Build history of the part. All positions in model axes, mm. Face numbers are marked on the shaded views. A direction names the side the tool comes from. Give positions to 0.01 mm unless a question says otherwise; leave off trailing zeros. Write each loop counter-clockwise with the first axis right and the second up, starting at its lowest first coordinate (ties: lowest second). Pieces come first, ordered by that corner, then holes.
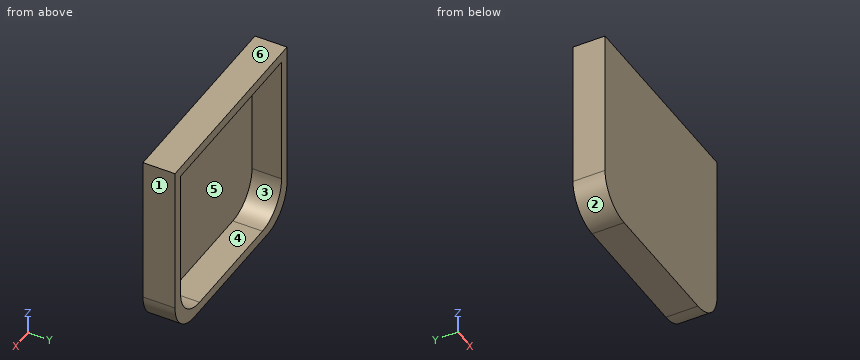
from build123d import *

# Parameters (mm, degrees)
BOSS_EXTRUDE1_DEPTH = 13
CUT_EXTRUDE1_DEPTH  = 12


with BuildPart() as part:
    # Sketch3 → Boss-Extrude1 (new body)
    with BuildSketch(Plane(origin=(0, 0, 0), x_dir=(1, 0, 0), z_dir=(0, 1, 0))):
        with BuildLine():
            Line((-41.015, -37.585), (41.015, -37.585))
            Line((41.015, -37.585), (41.015, 23.585))
            ThreePointArc((41.015, 23.585), (36.914494937, 33.484494937), (27.015, 37.585))
            Line((27.015, 37.585), (-27.015, 37.585))
            ThreePointArc((-27.015, 37.585), (-36.914494937, 33.484494937), (-41.015, 23.585))
            Line((-41.015, 23.585), (-41.015, -37.585))
        make_face()
    extrude(amount=BOSS_EXTRUDE1_DEPTH)

    # Sketch4 → Cut-Extrude1 (cut)
    with BuildSketch(Plane(origin=(0, 13, 0), x_dir=(1, 0, 0), z_dir=(0, 1, 0))):
        with BuildLine():
            Line((-37.015, -33.585), (37.015, -33.585))
            Line((37.015, -33.585), (37.015, 19.585))
            ThreePointArc((37.015, 19.585), (32.914494937, 29.484494937), (23.015, 33.585))
            Line((23.015, 33.585), (-23.015, 33.585))
            ThreePointArc((-23.015, 33.585), (-32.914494937, 29.484494937), (-37.015, 19.585))
            Line((-37.015, 19.585), (-37.015, -33.585))
        make_face()
    extrude(amount=-CUT_EXTRUDE1_DEPTH, mode=Mode.SUBTRACT)


solid = part.part
(1) Saw through at A-A, the plane y = 4.5. List the corners of the cut face in (x, z) (3 decimals), plus the area to 3 significant figures.
(2) Saw through at C-C, the plane z = 2. List the corners of the cut face in (x, y) (3 decimals), plus the area to 3 significant figures.
(3) 3-axis set-ups, long thin cutter, end or side, ignore diameter. For the marked faces 5 and 6: which of +Z, -Z, +X, -X, +Y, -Y reach the whole face in a straight line?
(4) Drop flat-ended pins along their axis: pin 1 (1 mm diameter, centred on x = 15.5, z = -13, fed in from -Y); pin 2 (3 mm diameter, centred on x = 2.5, z = -28, fed in from +Y); pin 3 (2 mm diameter, centred on x = 28.5, y = 10.5, fed in from -Z). Give the stop position or say it passes through.
(5) Mould opens along X. For the marked faces 1, 2, 3 and 4 say: +X half, -X half, draft (parallel to the pull), parting line (faces both ways), or undercut.
(6) Saw through at B-B, the plane x = -10. List the corners of the cut face in (y, z) (3 decimals), plus the area to 3 significant figures.
(7) Probe line 1 (Z direction, x = -15, y = 2) (3 decimals); line 2 (X direction, y = 10.25, z = -8.5) (3 decimals); line 3 (Y direction, x = 6, z = -11.5). List the from-to ranges inside material, lowest first.
Computed values:
1. outline: (-41.015, -23.585) arc R14 ccw to (-27.015, -37.585) - (27.015, -37.585) arc R14 ccw to (41.015, -23.585) - (41.015, 37.585) - (-41.015, 37.585) - close; hole (-37.015, -19.585) arc R14 ccw to (-23.015, -33.585) - (23.015, -33.585) arc R14 ccw to (37.015, -19.585) - (37.015, 33.585) - (-37.015, 33.585) - close
1. area: 1,190 mm2
2. outline: (-41.015, 0) - (41.015, 0) - (41.015, 13) - (37.015, 13) - (37.015, 1) - (-37.015, 1) - (-37.015, 13) - (-41.015, 13) - close
2. area: 178 mm2
3. face 5: +Y
3. face 6: +Z, +X, -X, +Y, -Y
4. pin 1: stops at y = 0
4. pin 2: stops at y = 1
4. pin 3: stops at z = -37.58
5. face 1: +X half
5. face 2: -X half
5. face 3: undercut
5. face 4: undercut
6. outline: (0, -37.585) - (13, -37.585) - (13, -33.585) - (1, -33.585) - (1, 33.585) - (13, 33.585) - (13, 37.585) - (0, 37.585) - close
6. area: 171 mm2
7. line 1: z = -37.585 to -33.585, 33.585 to 37.585
7. line 2: x = -41.015 to -37.015, 37.015 to 41.015
7. line 3: y = 0 to 1
